Verification items for the finished model (mm, model axes). Give positions to 0.01 mm unless a question says otherwise; leave off trailing zeros. Order: outer loops, then holes, each group sorted by start corner. A loop starts at its lowest first (then second) coordinate and runs counter-clockwise, first axis right, second up.
(1) Gauge pin test, flat ends, axial feed: pin 1 (8 mm diameter, centred on x = 97.5, y = 59, fed in from +Z); pin 2 (3 mm diameter, centred on y = 42.5, z = 1.5, fed in from -X); pin 3 (2 mm diameter, centred on x = 55.5, z = 2, fed in from +Y); pin 4 (2.5 mm diameter, centred on y = 2.5, z = 3.5, fed in from +X). Record the tip position at first contact, or that the pin passes through.
(2) Sectioned sample at A-A on y = 46.5. Record the cut outline in (x, z).
(3) Sectioned sample at D-D on z = 2.25. Count the separate pieces of the cut face and the enclosed holes in it, plus the area to 3 significant figures.
(4) Sectioned sample at C-C on y = 17.5. Record the cut outline in (x, z).
(5) Scan lines: L1, parallel to X at y = 14.5, z = 4.25; L2, parallel to Y at x = 57, z = 6; L3, parallel to X at y = 38.5, z = 0.75. Record each from-to range of solid material in increasing order.
(6) Sectioned sample at B-B on x = 33. Record the cut outline in (y, z) (3 decimals), plus the area to 3 significant figures.
```python
from build123d import *

# Parameters (mm, degrees)
SKETCH1_R           = 3.25
SKETCH1_R_2         = 1.1811
SKETCH1_W           = 6.858
SKETCH1_H           = 15
BOSS_EXTRUDE1_DEPTH = 6.92


with BuildPart() as part:
    # Sketch1 → Boss-Extrude1 (new body)
    with BuildSketch(Plane.XY):
        with BuildLine():
            Line((114.858, 9.999999315), (114.858, 49.5))
            ThreePointArc((114.858, 49.5), (114.779695723, 49.768649804), (114.569309131, 49.953153894))
            Line((114.569309131, 49.953153894), (67.125854783, 72.07639994))
            ThreePointArc((67.125854783, 72.07639994), (64.246101174, 71.887650915), (62.858, 69.357476578))
            Line((62.858, 69.357476578), (62.858, 38.83025734))
            ThreePointArc((62.858, 38.83025734), (62.049059599, 35.944627537), (59.858, 33.9))
            Line((59.858, 33.9), (59.858, 30.9))
            Line((59.858, 30.9), (53.098, 30.9))
            Line((53.098, 30.9), (53.098, 36.908691499))
            ThreePointArc((53.098, 36.908691499), (52.773590208, 37.645968836), (52.010844257, 37.904886197))
            Line((52.010844257, 37.904886197), (2.738532772, 33.594117516))
            ThreePointArc((2.738532772, 33.594117516), (0.78816799, 32.632304045), (0, 30.605533422))
            Line((0, 30.605533422), (0, 1))
            ThreePointArc((0, 1), (0.292893219, 0.292893219), (1, 0))
            Line((1, 0), (52.598, 0))
            ThreePointArc((52.598, 0), (52.951553391, 0.146446609), (53.098, 0.5))
            Line((53.098, 0.5), (53.098, 3.5))
            Line((53.098, 3.5), (59.858, 3.5))
            Line((59.858, 3.5), (59.858, 0.5))
            ThreePointArc((59.858, 0.5), (60.004446609, 0.146446609), (60.358, 0))
            Line((60.358, 0), (104.858, 0))
            ThreePointArc((104.858, 0), (111.92906757, 2.928931946), (114.858, 9.999999315))
        make_face()
        with Locations((65.858, 15.75)):
            Circle(SKETCH1_R, mode=Mode.SUBTRACT)
        with Locations((105.858, 15.75)):
            Circle(SKETCH1_R, mode=Mode.SUBTRACT)
        with Locations((109.858, 37.1528)):
            Circle(SKETCH1_R_2, mode=Mode.SUBTRACT)
        with Locations((109.858, 46.5)):
            Circle(SKETCH1_R_2, mode=Mode.SUBTRACT)
        with BuildLine():
            Line((50.108, 27.95), (50.108, 25.55))
            ThreePointArc((50.108, 25.55), (49.358, 24.8), (48.608, 25.55))
            Line((48.608, 25.55), (48.608, 27.95))
            ThreePointArc((48.608, 27.95), (49.358, 28.7), (50.108, 27.95))
        make_face(mode=Mode.SUBTRACT)
        with BuildLine():
            Line((43.108, 27.95), (43.108, 25.55))
            ThreePointArc((43.108, 25.55), (42.358, 24.8), (41.608, 25.55))
            Line((41.608, 25.55), (41.608, 27.95))
            ThreePointArc((41.608, 27.95), (42.358, 28.7), (43.108, 27.95))
        make_face(mode=Mode.SUBTRACT)
        with BuildLine():
            Line((35.858, 15.725), (27.858, 15.725))
            ThreePointArc((27.858, 15.725), (26.083, 17.5), (27.858, 19.275))
            Line((27.858, 19.275), (35.858, 19.275))
            ThreePointArc((35.858, 19.275), (37.633, 17.5), (35.858, 15.725))
        make_face(mode=Mode.SUBTRACT)
        with Locations((6.429, 21.084021409)):
            Rectangle(SKETCH1_W, SKETCH1_H, mode=Mode.SUBTRACT)
    extrude(amount=BOSS_EXTRUDE1_DEPTH)


solid = part.part
```
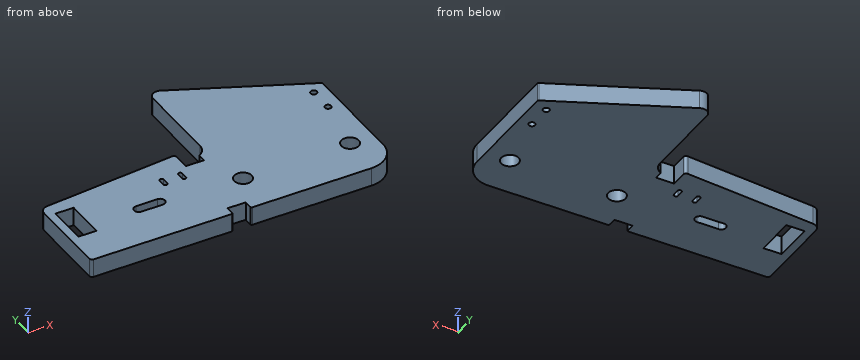
Ans:
1. pin 1: stops at z = 6.92
1. pin 2: stops at x = 62.86
1. pin 3: stops at y = 30.9
1. pin 4: stops at x = 112.66
2. outline: (62.86, 0) - (108.68, 0) - (108.68, 6.92) - (62.86, 6.92) - close; (111.04, 0) - (114.86, 0) - (114.86, 6.92) - (111.04, 6.92) - close
3. separate pieces: 1
3. enclosed holes: 8
3. area: 5,150 mm2
4. outline: (0, 0) - (3, 0) - (3, 6.92) - (0, 6.92) - close; (9.86, 0) - (26.08, 0) - (26.08, 6.92) - (9.86, 6.92) - close; (37.63, 0) - (63.12, 0) - (63.12, 6.92) - (37.63, 6.92) - close; (68.6, 0) - (103.12, 0) - (103.12, 6.92) - (68.6, 6.92) - close; (108.6, 0) - (114.86, 0) - (114.86, 6.92) - (108.6, 6.92) - close
5. L1: x = 0 to 3, 9.86 to 62.86, 68.86 to 102.86, 108.86 to 114.86
5. L2: y = 3.5 to 30.9
5. L3: x = 62.85 to 114.86
6. outline: (0, 0) - (15.725, 0) - (15.725, 6.92) - (0, 6.92) - close; (19.275, 0) - (36.242, 0) - (36.242, 6.92) - (19.275, 6.92) - close
6. area: 226 mm2
